```python
from build123d import *

# Parameters (mm, degrees)
SKETCH4_W           = 17
SKETCH4_H           = 11
BOSS_EXTRUDE2_DEPTH = 8.5
CUT_EXTRUDE1_DEPTH  = 13.5
CUT_EXTRUDE2_DEPTH  = 13.5
CUT_EXTRUDE3_DEPTH  = 13.5
CUT_EXTRUDE4_DEPTH  = 13.5
FILLET1_R           = 2
SKETCH16_W          = 45
SKETCH16_H          = 45
BOSS_EXTRUDE3_DEPTH = 10
SKETCH17_W          = 10
SKETCH17_H          = 35
BOSS_EXTRUDE4_DEPTH = 33.5
SKETCH18_W          = 15
SKETCH18_H          = 10
BOSS_EXTRUDE5_DEPTH = 22.5
SKETCH19_R          = 6
CUT_EXTRUDE5_DEPTH  = 28.5000001
FILLET3_R           = 10
FILLET4_R           = 20
SKETCH20_W          = 3
SKETCH20_H          = 8.5
BOSS_EXTRUDE6_DEPTH = 2.5
BOSS_EXTRUDE7_DEPTH = 3


with BuildPart() as part:
    # Sketch4 → Boss-Extrude2 (new body, symmetric)
    with BuildSketch(Plane.XY):
        Rectangle(SKETCH4_W, SKETCH4_H)
    extrude(amount=BOSS_EXTRUDE2_DEPTH, both=True)

    # Sketch5 → Cut-Extrude1 (cut, symmetric)
    with BuildSketch(Plane(origin=(0, 0, 0), x_dir=(0, 0, -1), z_dir=(1, 0, 0))):
        with BuildLine():
            Line((8.5, 5.5), (6.502509808, -1.291466653))
            ThreePointArc((6.502509808, -1.291466653), (6.473626767, -2.879228009), (7.259285969, -4.259285969))
            Line((7.259285969, -4.259285969), (8.5, -5.5))
            Line((8.5, -5.5), (8.5, 5.5))
        make_face()
        with BuildLine():
            Line((-8.5, -5.5), (-7.259285969, -4.259285969))
            ThreePointArc((-7.259285969, -4.259285969), (-6.473626767, -2.879228009), (-6.502509808, -1.291466653))
            Line((-6.502509808, -1.291466653), (-8.5, 5.5))
            Line((-8.5, 5.5), (-8.5, -5.5))
        make_face()
    extrude(amount=CUT_EXTRUDE1_DEPTH, both=True, mode=Mode.SUBTRACT)

    # Sketch7 → Cut-Extrude2 (cut, symmetric)
    with BuildSketch(Plane.XY):
        with BuildLine():
            Line((8.5, 5.5), (6.502538332, -1.291517059))
            ThreePointArc((6.502538332, -1.291517059), (6.473662442, -2.879270046), (7.259319467, -4.259319467))
            Line((7.259319467, -4.259319467), (8.5, -5.5))
            Line((8.5, -5.5), (8.5, 5.5))
        make_face()
        with BuildLine():
            Line((-8.5, -5.5), (-7.259319467, -4.259319467))
            ThreePointArc((-7.259319467, -4.259319467), (-6.473662442, -2.879270046), (-6.502538332, -1.291517059))
            Line((-6.502538332, -1.291517059), (-8.5, 5.5))
            Line((-8.5, 5.5), (-8.5, -5.5))
        make_face()
    extrude(amount=CUT_EXTRUDE2_DEPTH, both=True, mode=Mode.SUBTRACT)

    # Sketch11 → Cut-Extrude3 (cut, symmetric)
    with BuildSketch(Plane(origin=(0, 0, 0), x_dir=(0.707106781, 0, -0.707106781), z_dir=(0.707106781, 0, 0.707106781))):
        with BuildLine():
            Line((10, -5.5), (9.159523089, -4.659523089))
            ThreePointArc((9.159523089, -4.659523089), (8.341069319, -3.136306549), (8.499291869, -1.414382965))
            Line((8.499291869, -1.414382965), (9.693462893, 1.541294037))
            ThreePointArc((9.693462893, 1.541294037), (9.908907559, 2.799328578), (9.581873492, 4.033069244))
            ThreePointArc((9.581873492, 4.033069244), (9.013209006, 4.854851227), (8.25, 5.5))
            Line((8.25, 5.5), (14, 5.5))
            Line((14, 5.5), (14, -5.5))
            Line((14, -5.5), (10, -5.5))
        make_face()
        with BuildLine():
            Line((-14, 5.5), (-8.25, 5.5))
            ThreePointArc((-8.25, 5.5), (-9.013209006, 4.854851227), (-9.581873492, 4.033069244))
            ThreePointArc((-9.581873492, 4.033069244), (-9.908907559, 2.799328578), (-9.693462893, 1.541294037))
            Line((-9.693462893, 1.541294037), (-8.499291869, -1.414382965))
            ThreePointArc((-8.499291869, -1.414382965), (-8.341069319, -3.136306549), (-9.159523089, -4.659523089))
            Line((-9.159523089, -4.659523089), (-10, -5.5))
            Line((-10, -5.5), (-14, -5.5))
            Line((-14, -5.5), (-14, 5.5))
        make_face()
    extrude(amount=CUT_EXTRUDE3_DEPTH, both=True, mode=Mode.SUBTRACT)

    # Sketch12 → Cut-Extrude4 (cut, symmetric)
    with BuildSketch(Plane(origin=(0, 0, 0), x_dir=(-0.707106781, 0, -0.707106781), z_dir=(0.707106781, 0, -0.707106781))):
        with BuildLine():
            Line((10, -5.5), (9.159523089, -4.659523089))
            ThreePointArc((9.159523089, -4.659523089), (8.341069319, -3.136306549), (8.499291869, -1.414382965))
            Line((8.499291869, -1.414382965), (9.693462893, 1.541294037))
            ThreePointArc((9.693462893, 1.541294037), (9.908907559, 2.799328578), (9.581873492, 4.033069244))
            ThreePointArc((9.581873492, 4.033069244), (9.013209006, 4.854851227), (8.25, 5.5))
            Line((8.25, 5.5), (14, 5.5))
            Line((14, 5.5), (14, -5.5))
            Line((14, -5.5), (10, -5.5))
        make_face()
        with BuildLine():
            Line((-14, 5.5), (-8.25, 5.5))
            ThreePointArc((-8.25, 5.5), (-9.013209006, 4.854851227), (-9.581873492, 4.033069244))
            ThreePointArc((-9.581873492, 4.033069244), (-9.908907559, 2.799328578), (-9.693462893, 1.541294037))
            Line((-9.693462893, 1.541294037), (-8.499291869, -1.414382965))
            ThreePointArc((-8.499291869, -1.414382965), (-8.341069319, -3.136306549), (-9.159523089, -4.659523089))
            Line((-9.159523089, -4.659523089), (-10, -5.5))
            Line((-10, -5.5), (-14, -5.5))
            Line((-14, -5.5), (-14, 5.5))
        make_face()
    extrude(amount=CUT_EXTRUDE4_DEPTH, both=True, mode=Mode.SUBTRACT)

    # Sketch14 → Cut-Revolve1 (revolve, cut)
    with BuildSketch(Plane.XY):
        Polygon((0, 5.5), (5.5, 5.5), (2.5, 1.5), (2.5, -5.5), (0, -5.5), align=None)
    revolve(axis=Axis((0, -5.5, 0), (0, 1, 0)), mode=Mode.SUBTRACT)

    # Fillet1
    fillet1_edges = [part.edges().sort_by_distance(p)[0] for p in [
        (5.833630945, 5.5, -5.833630945),
        (-5.833630945, 5.5, -5.833630945),
        (-5.833630945, 5.5, 5.833630945),
        (5.833630945, 5.5, 5.833630945),
    ]]
    fillet(fillet1_edges, radius=FILLET1_R)

    # Sketch15 → Revolve1 (revolve)
    with BuildSketch(Plane(origin=(0, 0, 0), x_dir=(0, 0, -1), z_dir=(1, 0, 0))):
        with BuildLine():
            Line((0, -15.5), (22.5, -15.5))
            ThreePointArc((22.5, -15.5), (17.455904629, -8.920713416), (9.9979998, -5.3))
            Line((9.9979998, -5.3), (0, -5.3))
            Line((0, -5.3), (0, -5.5))
            Line((0, -5.5), (0, -15.5))
        make_face()
    revolve(axis=Axis((0, -5.5, 0), (0, -1, 0)))

    # Sketch16 → Boss-Extrude3 (add)
    with BuildSketch(Plane.XZ.offset(15.5)):
        Rectangle(SKETCH16_W, SKETCH16_H)
    extrude(amount=BOSS_EXTRUDE3_DEPTH)

    # Sketch17 → Boss-Extrude4 (add)
    with BuildSketch(Plane.XZ.offset(25.5)):
        with Locations((0, -5)):
            Rectangle(SKETCH17_W, SKETCH17_H)
    extrude(amount=BOSS_EXTRUDE4_DEPTH)

    # Sketch18 → Boss-Extrude5 (add)
    with BuildSketch(Plane.XZ.offset(25.5)):
        with Locations((15, 17.5)):
            Rectangle(SKETCH18_W, SKETCH18_H)
        with Locations((-15, 17.5)):
            Rectangle(SKETCH18_W, SKETCH18_H)
    extrude(amount=BOSS_EXTRUDE5_DEPTH)

    # Sketch19 → Cut-Extrude5 (cut, through all)
    with BuildSketch(Plane(origin=(5, 0, 0), x_dir=(0, 0, -1), z_dir=(1, 0, 0))):
        with Locations((-3.5, -48)):
            Circle(SKETCH19_R)
    extrude(amount=-CUT_EXTRUDE5_DEPTH, mode=Mode.SUBTRACT)

    # Fillet3
    fillet3_edges = [part.edges().sort_by_distance(p)[0] for p in [
        (-22.5, -31.75, 22.5),
        (22.5, -31.75, 22.5),
        (-22.5, -20.5, -22.5),
        (22.5, -20.5, -22.5),
        (0, -59, 12.5),
    ]]
    fillet(fillet3_edges, radius=FILLET3_R)

    # Fillet4
    fillet4_edges = [part.edges().sort_by_distance(p)[0] for p in [
        (0, -59, -22.5),
    ]]
    fillet(fillet4_edges, radius=FILLET4_R)

    # Sketch20 → Boss-Extrude6 (add)
    with BuildSketch(Plane.XY.offset(12.5)):
        with Locations((0, -29.75)):
            Rectangle(SKETCH20_W, SKETCH20_H)
    extrude(amount=BOSS_EXTRUDE6_DEPTH)

    # Sketch21 → Boss-Extrude7 (add)
    with BuildSketch(Plane(origin=(1.5, 0, 0), x_dir=(0, 0, -1), z_dir=(1, 0, 0))):
        Polygon((-15, -30.807466683), (-15, -34), (-21.577848346, -31.605858997), (-20.551787916, -28.786781134), align=None)
    extrude(amount=-BOSS_EXTRUDE7_DEPTH)


solid = part.part
```
Source: CAD feature listing. Evaluate the final solid. Frame: model axes, mm. A direction names the side the tool comes from. Coordinates: 2 decimals unless noted, no trailing zeros. Loops run counter-clockwise (first coordinate to the right, second up) from the corner with the lowest first, then second, coordinate; pieces in that order, holes last. Notation, with made-up numbers: M 16,63 L 22,63 A14 ccw 22,73 Z; hole C -9,49.25 d7. An arc over 180 degrees is marked long. Put each result on its own line as item: value. Start each with the question number.
1) Ray query, L1, parallel to Z at x = 0, y = -1.5; L2, parallel to X at y = -29.5, z = 3. Return the intervals inside material, ascending. Write a range as from..to.
2) Cut plane A-A on y = -24.5. Return the cut outline in (x, z), then the cut area to 3 significant figures.
3) Pull-direction query (X, two-part tool) for faces 5 (the face through (-0.34, 1.69, -2.62)), 6 (the face through (-4, 5.5, 4)), 7 (the face through (-5, -38, -5)); classes: pulls with the +X half, pulls with the -X half, needs draft (parallel to the pull), parting line crosses it, or undercut.
4) Contact query for flat-ended pins moving along their axis: pin 1 Ø18 at (x, z) = (16, 10.5) entering from +Y; pin 2 Ø17 at (y, z) = (-43.5, 0.5) entering from +X; pin 3 Ø1.2 at (x, z) = (0, 14) entering from -Y. Output: stop coordinate, or through.
5) Reachability of faces 1 (the face through (-15, -37, 12.5)), 2 (the face through (-6.43, 0.04, -6.42)), 3 (the face through (1.5, -31, 16)), 4 (the face through (0, -5.3, 0)) from +Z, -Z, +X, -X, +Y, -Y: full face, straight path, thin tool, end or side. Return the list, or none.
The answers:
1. L1: z = -6.45..-2.5, 2.5..6.45
1. L2: x = -5..5
2. outline: M -22.5,-12.5 A10 ccw -12.5,-22.5 L 12.5,-22.5 A10 ccw 22.5,-12.5 L 22.5,12.5 A10 ccw 12.5,22.5 L -12.5,22.5 A10 ccw -22.5,12.5 Z
2. area: 1,940 mm²
3. face 5: undercut
3. face 6: needs draft
3. face 7: pulls with the -X half
4. pin 1: stops at y = -5.33
4. pin 2: stops at x = 5
4. pin 3: stops at y = -34
5. face 1: -Z, -X, -Y
5. face 2: -Z, -X
5. face 3: +Z, -Y
5. face 4: +Y
